```python
from build123d import *

# Parameters (mm, degrees)
SKETCH1_W           = 29
SKETCH1_H           = 15.5
BOSS_EXTRUDE1_DEPTH = 1
BOSS_EXTRUDE2_DEPTH = 3.5
SKETCH4_W           = 5
SKETCH4_H           = 10
BOSS_EXTRUDE3_DEPTH = 3


with BuildPart() as part:
    # Sketch1 → Boss-Extrude1 (new body)
    with BuildSketch(Plane(origin=(0, 0, 0), x_dir=(1, 0, 0), z_dir=(0, 1, 0))):
        Rectangle(SKETCH1_W, SKETCH1_H)
    extrude(amount=BOSS_EXTRUDE1_DEPTH)

    # Sketch2 → Boss-Extrude2 (add)
    with BuildSketch(Plane(origin=(0, 1, 0), x_dir=(1, 0, 0), z_dir=(0, 1, 0))):
        with BuildLine():
            Line((-7, -3), (-0.5, -3))
            ThreePointArc((-0.5, -3), (1.25, -4.75), (-0.5, -6.5))
            Line((-0.5, -6.5), (-7, -6.5))
            ThreePointArc((-7, -6.5), (-8.75, -4.75), (-7, -3))
        make_face()
    extrude(amount=BOSS_EXTRUDE2_DEPTH)

    # Sketch4 → Boss-Extrude3 (add)
    with BuildSketch(Plane.XZ):
        with Locations((-11.8, -2.25)):
            Rectangle(SKETCH4_W, SKETCH4_H)
    extrude(amount=BOSS_EXTRUDE3_DEPTH)


solid = part.part
```
Geometry: final body of the model. Coordinates: model frame, mm. A direction names the side the tool comes from. Coordinates: 2 decimals unless noted, no trailing zeros. Order: outer loops, then holes, each group sorted by start corner. A loop starts at its lowest first (then second) coordinate and runs counter-clockwise, first axis right, second up. Notation, with made-up numbers: (12, 60.25) - (16, 60.25) arc R15 ccw to (16, 66.25) - close; hole circle Ø6 at (46.25, 50). An arc over 180 degrees is marked (long way). Return JSON: item names as keys, results as strings. Group by question number.
1. Cut plane A-A (x = -10). Output: boundary loops of the cut face in (y, z), plus the area to 3 significant figures.
2. Pin query (flat end, axial travel): pin 1 (1 mm diameter, centred on x = -3, z = -1, fed in from -Y); pin 2 (1.5 mm diameter, centred on y = -1, z = -2, fed in from +X); pin 3 (3 mm diameter, centred on x = 9, z = 1.5, fed in from +Y). Return the tip coordinate at first contact, or that it passes through.
3. Cut plane D-D (x = 2). Output: boundary loops of the cut face in (y, z).
4. Set-up query: faces 1 (the face through (-4, 3, 6.5)), 2 (the face through (-4, 3, 3)), 3 (the face through (1.25, 2.73, 4.71)), 4 (the face through (-12, -1, -7.25)), 5 (the face through (-12, -1, 2.75)). Return all of +Z, -Z, +X, -X, +Y, -Y with unobstructed straight access to the full face (end or side cutting, diameter ignored); none if empty.
5. Cut plane C-C (y = 3.25). Output: boundary loops of the cut face in (x, z), plus the area to 3 significant figures.
6. Cut plane B-B (z = 4.75). Output: boundary loops of the cut face in (x, y), plus the area to 3 significant figures.
7. Material intervals for line 1 along Y through (x, z) = (-1, 7); line 2 along X through (y, z) = (-2.5, -4.75); line 3 along Y through (x, z) = (-9.75, -0.25), sorted ascending. Write a range as [from, to].
Resolved:
{
 "1": {"outline": "(-3, -7.25) - (0, -7.25) - (0, -7.75) - (1, -7.75) - (1, 7.75) - (0, 7.75) - (0, 2.75) - (-3, 2.75) - close", "area": "45.5 mm²"},
 "2": {"pin 1": "stops at y = 0", "pin 2": "stops at x = -9.3", "pin 3": "stops at y = 1"},
 "3": {"outline": "(0, -7.75) - (1, -7.75) - (1, 7.75) - (0, 7.75) - close"},
 "4": {"face 1": "+Z, +X, -X, +Y", "face 2": "-Z, +X, -X, +Y", "face 3": "+X, +Y", "face 4": "-Z, +X, -X, -Y", "face 5": "+Z, +X, -X, -Y"},
 "5": {"outline": "(-7, 3) - (-0.5, 3) arc R1.75 ccw to (-0.5, 6.5) - (-7, 6.5) arc R1.75 ccw to start", "area": "32.4 mm²"},
 "6": {"outline": "(-14.5, 0) - (14.5, 0) - (14.5, 1) - (1.25, 1) - (1.25, 4.5) - (-8.75, 4.5) - (-8.75, 1) - (-14.5, 1) - close", "area": "64.0 mm²"},
 "7": {"line 1": "y = [0, 1]", "line 2": "x = [-14.3, -9.3]", "line 3": "y = [-3, 1]"}
}
